Autodesk Inventor part; units mm, degrees
ref_plane "YZ Plane" through (0, 0, 0) normal (1, 0, 0) x (0, 1, 0)
ref_plane "XZ Plane" through (0, 0, 0) normal (0, 1, 0) x (-1, 0, 0)
ref_plane "XY Plane" through (0, 0, 0) normal (0, 0, 1) x (1, 0, 0)
sketch "Esquisse1" plane through (0, 0, 0) normal (0, 1, 0) x (-1, 0, 0)
  line L0 (6.15, 11.25) -> (-6.15, 11.25)
  line L1 (-6.15, 11.25) -> (-6.15, -11.25)
  line L2 (-6.15, -11.25) -> (6.15, -11.25)
  line L3 (6.15, -11.25) -> (6.15, 11.25)
  line L4 (6.15, 11.25) -> (-6.15, -11.25)
  line L5 (-6.15, 11.25) -> (6.15, -11.25)
  point P0 (0, 0)
  point P1 (0, 0)
  point P2 (0, 0)
  dimension "d0" = 22.5
  dimension "d1" = 12.3
extrude "Extrusion1" add sketch "Esquisse1" along normal blind 22.6
sketch "Esquisse2" plane through (-6.15, 0, 11.25) normal (0, 0, 1) x (1, 0, 0)
  line L0 (0, 0) -> (0, 22.6)
  line L1 (12.3, 0) -> (12.3, 22.6)
  line L2 (0, 18.4) -> (12.3, 18.4)
  line L3 (12.3, 18.4) -> (12.3, 16.1)
  line L4 (12.3, 16.1) -> (0, 16.1)
  line L5 (0, 16.1) -> (0, 18.4)
  line L6 (0, 0) -> (12.3, 0)
  point P0 (6.15, 0)
  point P1 (0, 16.1)
  dimension "d4" = 2.3
  dimension "d5" = 16.1
extrude "Extrusion2" add sketch "Esquisse2" along normal blind 6 contours L0 L2 L1 L4
sketch "Esquisse3" plane through (6.15, 0, -11.25) normal (0, 0, -1) x (-1, 0, 0)
  line L0 (12.3, 18.4) -> (0, 18.4)
  line L1 (12.3, 0) -> (12.3, 16.1)
  line L2 (0, 18.4) -> (12.3, 18.4)
  line L3 (12.3, 18.4) -> (12.3, 16.1)
  line L4 (12.3, 16.1) -> (0, 16.1)
  line L5 (0, 16.1) -> (0, 18.4)
  point P0 (6.15, 0)
extrude "Extrusion3" add sketch "Esquisse3" along normal blind 6
sketch "Esquisse4" plane through (0, 22.6, 0) normal (0, 1, 0) x (1, 0, 0)
  circle A0 centre (0, -5.1) radius 6.15
  line L0 (-6.15, 11.25) -> (-6.15, -11.25)
  line L1 (-6.15, -11.25) -> (6.15, -11.25)
  circle A1 centre (0, 0.6) radius 2.75
  point P0 (0, 0)
  point P1 (-2.743, 0.4044)
  point P2 (2.743, 0.4044)
  dimension "d10" = 12.3
  dimension "d11" = 6.15
  dimension "d12" = 5.5
  dimension "d13" = 14.6
extrude "Extrusion4" add sketch "Esquisse4" along normal blind 5 contours A0 A1 | A1 A0 | A0 A1
sketch "Esquisse5" plane through (0, 27.6, 0) normal (0, 1, 0) x (1, 0, 0)
  arc A0 (-6.15, -5.1) -> (0, -11.25) centre (0, -5.1) ccw
  circle A1 centre (0, -5.1) radius 2.4
  point P0 (0, 0)
  dimension "d16" = 4.8
extrude "Extrusion5" add sketch "Esquisse5" along normal blind 3.7
properties part number "servomoteur"
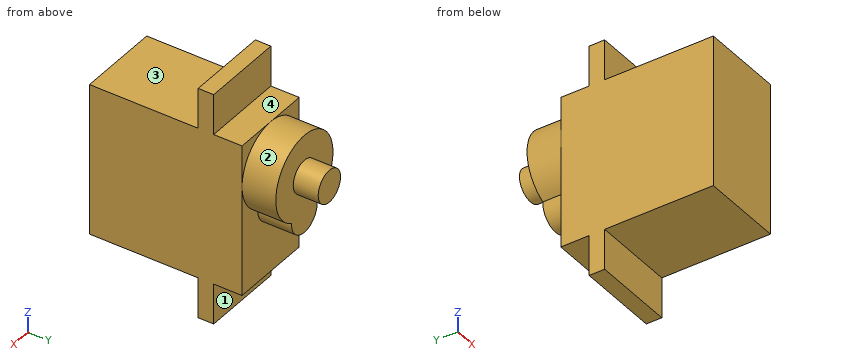
Check sheet for the modelled part. Datum: model origin and axes. Units: mm. Face numbers are marked on the shaded views. A direction names the side the tool comes from. Give positions to 0.01 mm unless a question says otherwise; leave off trailing zeros. Loops run counter-clockwise (first coordinate to the right, second up) from the corner with the lowest first, then second, coordinate; pieces in that order, holes last. Notation, with made-up numbers: M -25.75,52 L 6.25,52 A10 cw 6.25,64 Z; hole C 26,2.5 d2. An arc over 180 degrees is marked long. Use a Markdown table: item, result. Add a question column.
Q1. Tool access check on the marked faces 1, 2, 3 and 4. Record the directions out of +Z, -Z, +X, -X, +Y, -Y that give a thin tool (end or side, any length) a straight path to the whole face; none if there is none.
Q2. Sectioned sample at A-A, the plane x = -4.75. Record the cut outline in (y, z).
Q3. Sectioned sample at C-C, the plane y = 3. Record the cut outline in (x, z), then the cut area to 3 significant figures.
Q4. Scan lines: line 1 along Z through (x, y) = (-4.5, 21); line 2 along Y through (x, z) = (1.25, 12); line 3 along Y through (x, z) = (3.75, -8). Record each from-to range of solid material in increasing order. Write a range as [from, to].
Q5. Sectioned sample at D-D, the plane x = 1.5. Record the cut outline in (y, z), then the cut area to 3 significant figures.
Q6. Go/stop test with flat-tipped pins: pin 1 (3.5 mm diameter, centred on x = -1, z = -1, fed in from +Y); pin 2 (3 mm diameter, centred on x = 1.5, z = -14.5, fed in from +Y); pin 3 (3.5 mm diameter, centred on x = -3, y = 21.5, fed in from -Z). Record where each tip stops, or that it passes through.
Q7. Sectioned sample at B-B, the plane z = -12. Record the cut outline in (x, y).
Verdict:
| question | item | result |
|---|---|---|
| 1 | face 1 | -Z, +X, -X, +Y |
| 1 | face 2 | +Y |
| 1 | face 3 | +Z, +X, -X, -Y |
| 1 | face 4 | +Z, +X, -X, +Y |
| 2 | outline | M 0,-11.25 L 16.1,-11.25 L 16.1,-17.25 L 18.4,-17.25 L 18.4,-11.25 L 22.6,-11.25 L 22.6,1.19 L 27.6,1.19 L 27.6,9.01 L 22.6,9.01 L 22.6,11.25 L 18.4,11.25 L 18.4,17.25 L 16.1,17.25 L 16.1,11.25 L 0,11.25 Z |
| 3 | outline | M -6.15,-11.25 L 6.15,-11.25 L 6.15,11.25 L -6.15,11.25 Z |
| 3 | area | 277 mm^2 |
| 4 | line 1 | [-11.25, 11.25] |
| 4 | line 2 | [16.1, 18.4] |
| 4 | line 3 | [0, 22.6] |
| 5 | outline | M 0,-11.25 L 16.1,-11.25 L 16.1,-17.25 L 18.4,-17.25 L 18.4,-11.25 L 22.6,-11.25 L 22.6,-2.9 L 27.6,-2.9 L 27.6,3.23 L 31.3,3.23 L 31.3,6.97 L 27.6,6.97 L 27.6,11.06 L 22.6,11.06 L 22.6,11.25 L 18.4,11.25 L 18.4,17.25 L 16.1,17.25 L 16.1,11.25 L 0,11.25 Z |
| 5 | area | 620 mm^2 |
| 6 | pin 1 | y = 27.6 |
| 6 | pin 2 | y = 18.4 |
| 6 | pin 3 | z = -11.25 |
| 7 | outline | M -6.15,16.1 L 6.15,16.1 L 6.15,18.4 L -6.15,18.4 Z |
